For this review, take the finished solid that the model builds, in its own axes (mm). Face numbers are marked on the shaded views. Give positions to 0.01 mm unless a question says otherwise; leave off trailing zeros. Loops run counter-clockwise (first coordinate to the right, second up) from the corner with the lowest first, then second, coordinate; pieces in that order, holes last.
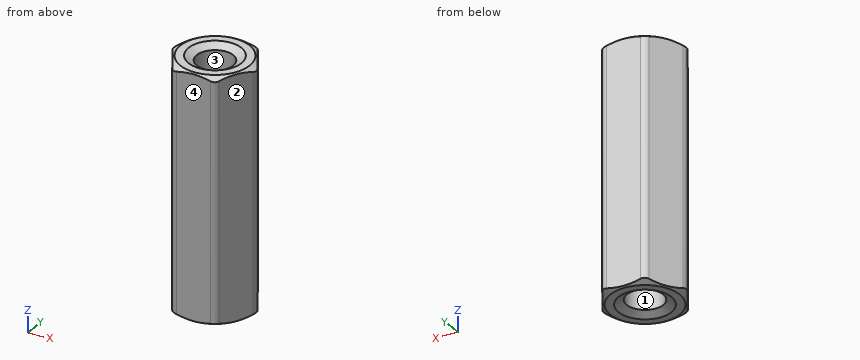
```python
from build123d import *

# Parameters (mm, degrees)
SKETCH4_R           = 2.25
BOSS_EXTRUDE1_DEPTH = 10
SKETCH5_OUTSIDE_W   = 87.87
SKETCH5_OUTSIDE_H   = 86.942
SKETCH5_OUTSIDE_R   = 2.85
CUT_EXTRUDE1_DEPTH  = 21.518284529
CUT_EXTRUDE1_DRAFT  = -60
SKETCH6_OUTSIDE_W   = 87.87
SKETCH6_OUTSIDE_H   = 86.942
SKETCH6_OUTSIDE_R   = 2.85
CUT_EXTRUDE2_DEPTH  = 21.518284529
CUT_EXTRUDE2_DRAFT  = -60
FILLET1_R           = 0.6
BOSS_EXTRUDE2_START = -10
SKETCH7_R           = 2.175
BOSS_EXTRUDE2_DEPTH = 6.3
SKETCH8_W           = 6.3
SKETCH8_H           = 1.5
CIRPATTERN1_COUNT   = 2


with BuildPart() as part:
    # Sketch3 → Revolve1 (revolve)
    with BuildSketch(Plane(origin=(0, 0, 0), x_dir=(0, 0, -1), z_dir=(1, 0, 0))):
        Polygon((-9.610288568, 1.5), (-3.7, 1.5), (-3.7, 0), (3.7, 0), (3.7, 1.5), (9.610288568, 1.5), (10, 2.175), (10, 3), (0, 3), (-10, 3), (-10, 2.175), align=None)
        Polygon((-9.610288568, 1.5), (-3.7, 1.5), (-3.7, 0), (3.7, 0), (3.7, 1.5), (9.610288568, 1.5), (10, 2.175), (10, 3), (0, 3), (-10, 3), (-10, 2.175), align=None)
    revolve(axis=Axis((0, 0, 3.7), (0, 0, 1)))

    # Sketch4 → Boss-Extrude1 (add, symmetric)
    with BuildSketch(Plane.XY):
        Polygon((-1.732050808, 3), (-3.464101615, 0), (-1.732050808, -3), (1.732050808, -3), (3.464101615, 0), (1.732050808, 3), align=None)
        Circle(SKETCH4_R, mode=Mode.SUBTRACT)
    extrude(amount=BOSS_EXTRUDE1_DEPTH, both=True)


with BuildPart() as cut_extrude1_tool:
    # Sketch5 outside → Cut-Extrude1 (with draft: the straight prism first)
    with BuildSketch(Plane.XY.offset(10)):
        Rectangle(SKETCH5_OUTSIDE_W, SKETCH5_OUTSIDE_H)
        Circle(SKETCH5_OUTSIDE_R, mode=Mode.SUBTRACT)
    extrude(amount=-CUT_EXTRUDE1_DEPTH)
    # Cut-Extrude1: the draft: its side faces are tilted about the plane it starts from
    cut_extrude1_sides = [cut_extrude1_tool.faces().sort_by_distance(p)[0] for p in [
        (0, -43.471, -0.759142264),
        (43.935, 0, -0.759142264),
        (0, 43.471, -0.759142264),
        (-43.935, 0, -0.759142264),
        (-2.85, 0, -0.759142264),
    ]]
    draft(cut_extrude1_sides, Plane.XY.offset(10), CUT_EXTRUDE1_DRAFT)


with BuildPart() as part_1:
    add(part.part)

    # Cut-Extrude1: cut by cut_extrude1_tool
    add(cut_extrude1_tool.part, mode=Mode.SUBTRACT)


with BuildPart() as cut_extrude2_tool:
    # Sketch6 outside → Cut-Extrude2 (with draft: the straight prism first)
    with BuildSketch(Plane(origin=(0, 0, -10), x_dir=(-1, 0, 0), z_dir=(0, 0, -1))):
        Rectangle(SKETCH6_OUTSIDE_W, SKETCH6_OUTSIDE_H)
        Circle(SKETCH6_OUTSIDE_R, mode=Mode.SUBTRACT)
    extrude(amount=-CUT_EXTRUDE2_DEPTH)
    # Cut-Extrude2: the draft: its side faces are tilted about the plane it starts from
    cut_extrude2_sides = [cut_extrude2_tool.faces().sort_by_distance(p)[0] for p in [
        (0, -43.471, 0.759142264),
        (-43.935, 0, 0.759142264),
        (0, 43.471, 0.759142264),
        (43.935, 0, 0.759142264),
        (2.85, 0, 0.759142264),
    ]]
    draft(cut_extrude2_sides, Plane(origin=(0, 0, -10), x_dir=(-1, 0, 0), z_dir=(0, 0, -1)), CUT_EXTRUDE2_DRAFT)


with BuildPart() as part_2:
    add(part_1.part)

    # Cut-Extrude2: cut by cut_extrude2_tool
    add(cut_extrude2_tool.part, mode=Mode.SUBTRACT)

    # Fillet1
    # the kernel refuses this fillet: 0.6 mm, written as the material it takes off along each edge
    with BuildSketch(Plane(origin=(1.732050808, 3, 10.511473671), x_dir=(-1, 0, 0), z_dir=(0, 0, -1)), Plane(origin=(-1.732050808, 3, 10.511473671), x_dir=(-0.5000000000000006, -0.8660254037844383, 0), z_dir=(0, 0, -1))) as fillet1_piece_1:
        with BuildLine():
            CenterArc((FILLET1_R * 0.57735026919, -FILLET1_R), FILLET1_R, 90, 60)
            Line((-FILLET1_R * 0.288675134595, -FILLET1_R * 0.5), (0, 0))
            Line((0, 0), (FILLET1_R * 0.57735026919, 0))
        make_face()
    extrude(amount=21.022947342, mode=Mode.SUBTRACT)
    with BuildSketch(Plane(origin=(-3.464101615, 0, -10.511473671), x_dir=(0.5000000000000008, -0.8660254037844383, 0), z_dir=(0, 0, 1)), Plane(origin=(-1.732050808, -3, -10.511473671), x_dir=(1, 0, 0), z_dir=(0, 0, 1)), Plane(origin=(1.732050808, -3, -10.511473671), x_dir=(0.5000000000000001, 0.8660254037844386, 0), z_dir=(0, 0, 1)), Plane(origin=(3.464101615, 0, 10.511473671), x_dir=(-0.4999999999999995, -0.8660254037844388, 0), z_dir=(0, 0, -1))) as fillet1_piece_2:
        with BuildLine():
            CenterArc((FILLET1_R * 0.57735026919, FILLET1_R), FILLET1_R, 210, 60)
            Line((-FILLET1_R * 0.288675134595, FILLET1_R * 0.5), (0, 0))
            Line((0, 0), (FILLET1_R * 0.57735026919, 0))
        make_face()
    extrude(amount=21.022947342, mode=Mode.SUBTRACT)

    # Sketch7 → Boss-Extrude2 (add)
    with BuildSketch(Plane(origin=(0, 0, 0), x_dir=(-1, 0, 0), z_dir=(0, 0, -1)).offset(BOSS_EXTRUDE2_START)):
        Circle(SKETCH7_R)
    extrude(amount=BOSS_EXTRUDE2_DEPTH)

    # SurfaceCut1
    split(bisect_by=Plane.XY, keep=Keep.TOP)


with BuildPart() as body_2:
    # Sketch8 → Revolve2 (revolve)
    with BuildSketch(Plane(origin=(0, 0, 0), x_dir=(0, 0, -1), z_dir=(1, 0, 0))):
        with Locations((-6.85, 0.75)):
            Rectangle(SKETCH8_W, SKETCH8_H)
    revolve(axis=Axis((0, 0, 3.7), (0, 0, 1)))


with BuildPart() as part_3:
    add(part_2.part)

    # Combine1: cut body 2
    add(body_2.part, mode=Mode.SUBTRACT)

    # Cut-Extrude3 cone 1 section (through the dimple's axis) → Cut-Extrude3 (revolve, cut)
    with BuildSketch(Plane(origin=(0, 0, 10), x_dir=(0, -1, 0), z_dir=(1, 0, 0))):
        Polygon((0, 0), (2.175, 0), (0, 1.255736835), align=None)
    revolve(axis=Axis((0, 0, 10), (0, 0, -1)), mode=Mode.SUBTRACT)


with BuildPart() as cirpattern1_1:
    # CirPattern1: pattern copy
    add(part_3.part.rotate(Axis((0, 0, 0), (1, 0, 0)), 1 * 360 / CIRPATTERN1_COUNT))


with BuildPart() as part_4:
    add(part_3.part)

    # Combine2: union CirPattern1_1
    add(cirpattern1_1.part)


solid = part_4.part
```
Q1. Consider section C-C on x = 0. Give the boundary of the cut face in (y, z) (3 decimals).
Answers:
outline: (-3, -9.913) - (-2.85, -10) - (-2.175, -10) - (-1.5, -9.61) - (-1.5, -3.7) - (1.5, -3.7) - (1.5, -9.61) - (2.175, -10) - (2.85, -10) - (3, -9.913) - (3, 9.913) - (2.85, 10) - (2.175, 10) - (1.5, 9.61) - (1.5, 3.7) - (-1.5, 3.7) - (-1.5, 9.61) - (-2.175, 10) - (-2.85, 10) - (-3, 9.913) - close
Q2. Consider section A-A on y = 0. Give the boundary of the cut face in (x, z) (3 decimals).
Answers:
outline: (-3.371, -9.699) - (-2.85, -10) - (-2.175, -10) - (-1.5, -9.61) - (-1.5, -3.7) - (1.5, -3.7) - (1.5, -9.61) - (2.175, -10) - (2.85, -10) - (3.371, -9.699) - (3.371, 9.699) - (2.85, 10) - (2.175, 10) - (1.5, 9.61) - (1.5, 3.7) - (-1.5, 3.7) - (-1.5, 9.61) - (-2.175, 10) - (-2.85, 10) - (-3.371, 9.699) - close
Q3. Consider section B-B on z = 4.5. Give the boundary of the cut face in (x, y).
Answers:
outline: (-3.29, -0.3) - (-1.91, -2.7) arc R0.6 ccw to (-1.39, -3) - (1.39, -3) arc R0.6 ccw to (1.91, -2.7) - (3.29, -0.3) arc R0.6 ccw to (3.29, 0.3) - (1.91, 2.7) arc R0.6 ccw to (1.39, 3) - (-1.39, 3) arc R0.6 ccw to (-1.91, 2.7) - (-3.29, 0.3) arc R0.6 ccw to start; hole circle Ø3 at (0, 0)
Q4. Consider section D-D on z = 1. Give the boundary of the cut face in (x, y).
Answers:
outline: (-3.29, -0.3) - (-1.91, -2.7) arc R0.6 ccw to (-1.39, -3) - (1.39, -3) arc R0.6 ccw to (1.91, -2.7) - (3.29, -0.3) arc R0.6 ccw to (3.29, 0.3) - (1.91, 2.7) arc R0.6 ccw to (1.39, 3) - (-1.39, 3) arc R0.6 ccw to (-1.91, 2.7) - (-3.29, 0.3) arc R0.6 ccw to start
Q5. Mouldability with a two-part tool opening along X and no side actions: class the marked faces 1, 2, 3 and 4 as +X half, -X half, draft (parallel to the pull), parting line (faces both ways), or undercut.
Answers:
face 1: undercut
face 2: +X half
face 3: undercut
face 4: draft
Q6. For probe 1 along X at (y, z) = (0, 8.3); probe 2 along Y at (x, z) = (0, 6.75); probe 3 along Z at (x, y) = (-0.75, 0.25), list the stretches that pass through material, from the lowest coordinate up.
Answers:
probe 1: x = -3.37 to -1.5, 1.5 to 3.37
probe 2: y = -3 to -1.5, 1.5 to 3
probe 3: z = -3.7 to 3.7
Q7. For pin 1 Ø0.9 at (x, y) = (-0.5, 0.5) entering from +Z; pin 2 Ø2.5 at (x, y) = (0.5, -0.5) entering from -Z, all flat-tipped, find the tip position at first contact; note any pin that passes through.
Answers:
pin 1: stops at z = 3.7
pin 2: stops at z = -9.87
